```python
from build123d import *

# Parameters (mm, degrees)
PAD_DEPTH     = 15
SKETCH001_R   = 2
POCKET_DEPTH  = 6.951
SKETCH003_R   = 1
PAD001_DEPTH  = 9
SKETCH004_W   = 4.5
SKETCH004_H   = 4.5
SKETCH004_W_2 = 3.5
SKETCH004_H_2 = 3.5
PAD002_DEPTH  = 24
SKETCH008_W   = 3
SKETCH008_H   = 10
PAD005_DEPTH  = 7.2
SKETCH009_W   = 27
SKETCH009_H   = 10
PAD006_DEPTH  = 2


with BuildPart() as part:
    # Sketch → Pad (new body)
    with BuildSketch(Plane.YZ):
        Polygon((0, 0), (7.355, 0), (7.355, -2.25), (4.955, -2.25), (4.955, -3.25), (7.355, -5.75), (12.855, -5.75), (15.255, -3.25), (15.255, -2.25), (12.855, -2.25), (12.855, 0), (80, 0), (80, 1.2), (0, 1.2), align=None)
    extrude(amount=PAD_DEPTH)

    # Sketch001 (on Face13 of Pad) → Pocket (cut, through all)
    with BuildSketch(Plane(origin=(0, 0, 1.2), x_dir=(0, -1, 0), z_dir=(0, 0, 1))):
        with Locations((-70, 5)):
            Circle(SKETCH001_R)
    extrude(amount=-POCKET_DEPTH, mode=Mode.SUBTRACT)

    # Sketch003 (on Face6 of Pocket) → Pad001 (join)
    with BuildSketch(Plane(origin=(0, 0, 1.2), x_dir=(0, -1, 0), z_dir=(0, 0, 1))):
        with Locations((-43.5, 7.5)):
            Circle(SKETCH003_R)
        with Locations((-34, 7.5)):
            Circle(SKETCH003_R)
    extrude(amount=PAD001_DEPTH)

    # Sketch004 → Pad002 (join)
    with BuildSketch(Plane.XZ):
        with Locations((2.25, 3.45)):
            Rectangle(SKETCH004_W, SKETCH004_H)
        with Locations((2.25, 3.45)):
            Rectangle(SKETCH004_W_2, SKETCH004_H_2, mode=Mode.SUBTRACT)
    extrude(amount=-PAD002_DEPTH)

    # Sketch008 (on Face6 of Pad002) → Pad005 (join)
    with BuildSketch(Plane(origin=(0, 0, 1.2), x_dir=(0, -1, 0), z_dir=(0, 0, 1))):
        with Locations((-51.1, 10)):
            Rectangle(SKETCH008_W, SKETCH008_H)
        with Locations((-27.1, 10)):
            Rectangle(SKETCH008_W, SKETCH008_H)
    extrude(amount=PAD005_DEPTH)

    # Sketch009 (on Face32 of Pad005) → Pad006 (join)
    with BuildSketch(Plane(origin=(0, 0, 8.4), x_dir=(0, -1, 0), z_dir=(0, 0, 1))):
        with Locations((-39.1, 10)):
            Rectangle(SKETCH009_W, SKETCH009_H)
    extrude(amount=PAD006_DEPTH)


solid = part.part
```
Build history of the part. All positions in model axes, mm. A direction names the side the tool comes from. Give positions to 0.01 mm unless a question says otherwise; leave off trailing zeros. Order: outer loops, then holes, each group sorted by start corner. A loop starts at its lowest first (then second) coordinate and runs counter-clockwise, first axis right, second up. Notation, with made-up numbers: M 1,24.25 L 35,24.25 A28 ccw 35,52.25 Z; hole C 36.5,-2 d3. An arc over 180 degrees is marked long. Return JSON: item names as keys, results as strings.
Q1. Flat gauge pins, fed straight in: pin 1 (1.5 mm diameter, centred on x = 7, y = 26, fed in from -Z); pin 2 (5 mm diameter, centred on x = 2, y = 15.5, fed in from +Z); pin 3 (3.5 mm diameter, centred on y = 11.5, z = 4, fed in from +X). Where does each tip first touch, or does it go through?
Answer list:
{"pin 1": "stops at z = 0", "pin 2": "stops at z = 5.7", "pin 3": "stops at x = 4.5"}
Q2. Band-saw the part on C-C (z = 3.25). Give the cut face in (x, y).
Answer list:
{"outline": "M 0,0 L 0.5,0 L 0.5,24 L 0,24 Z; M 4,0 L 4.5,0 L 4.5,24 L 4,24 Z; M 5,25.6 L 15,25.6 L 15,28.6 L 5,28.6 Z; M 5,49.6 L 15,49.6 L 15,52.6 L 5,52.6 Z; C 7.5,34 d2; C 7.5,43.5 d2"}
Q3. Band-saw the part on D-D (y = 34). Give the cut face in (x, z).
Answer list:
{"outline": "M 0,0 L 15,0 L 15,1.2 L 8.5,1.2 L 8.5,8.4 L 15,8.4 L 15,10.4 L 5,10.4 L 5,8.4 L 6.5,8.4 L 6.5,1.2 L 0,1.2 Z"}
Q4. Band-saw the part on A-A (y = 70). Give the cut face in (x, z).
Answer list:
{"outline": "M 0,0 L 3,0 L 3,1.2 L 0,1.2 Z; M 7,0 L 15,0 L 15,1.2 L 7,1.2 Z"}
Q5. 3-axis set-ups, long thin cutter, end or side, ignore diameter. For faces 1 (the face through (7.8, 42.546, 4.75)), 2 (the face through (7, 7.355, -1)), 3 (the face through (2.2, 24, 1.5)), 4 (the face through (4, 12, 3)): which of +Z, -Z, +X, -X, +Y, -Y reach the whole face in a straight line?
Answer list:
{"face 1": "none", "face 2": "+X, -X, -Y", "face 3": "+Z, +X, -X, +Y", "face 4": "+Y, -Y"}
Q6. Two-plate mould, pull along Y, no slides. Class faces 5 (the face through (10, 28.6, 5)), 6 (the face through (10, 49.6, 5)), 7 (the face through (2, 12, 5.7)), 8 (the face through (10, 25.6, 6)): pulls with the +Y half, pulls with the -Y half, needs draft (parallel to the pull), parting line crosses it, or undercut.
Answer list:
{"face 5": "undercut", "face 6": "undercut", "face 7": "needs draft", "face 8": "pulls with the -Y half"}
Q7. Band-saw the part on B-B (z = 7). Give the cut face in (x, y).
Answer list:
{"outline": "M 5,25.6 L 15,25.6 L 15,28.6 L 5,28.6 Z; M 5,49.6 L 15,49.6 L 15,52.6 L 5,52.6 Z; C 7.5,34 d2; C 7.5,43.5 d2"}
Q8. Wall check: probe 1 along X at (y, z) = (70, 0.6); probe 2 along X at (y, z) = (10, 4.75); probe 3 along Z at (x, y) = (2.25, 15). Give the ranges that are in metal, low to high. Write a range as from..to.
Answer list:
{"probe 1": "x = 0..3, 7..15", "probe 2": "x = 0..0.5, 4..4.5", "probe 3": "z = -3.52..-2.25, 0..1.7, 5.2..5.7"}
